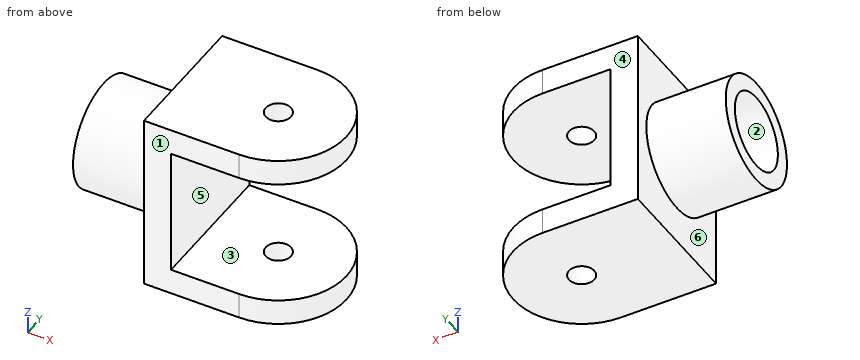
from build123d import *

# Parameters (mm, degrees)
BOSS_EXTRUDE2_DEPTH      = 11.35
BOSS_EXTRUDE2_DEPTH_BACK = 11.35
SKETCH1_R                = 1.5875
CUT_EXTRUDE1_DEPTH       = 8.08
CUT_EXTRUDE1_DEPTH_BACK  = 8.08
SKETCH3_W                = 17.175
SKETCH3_H                = 17.175
SKETCH4_R                = 6.7225
SKETCH4_R_2              = 4.7225
BOSS_EXTRUDE4_DEPTH      = 10


with BuildPart() as part:
    # Sketch1 → Boss-Extrude2 (new, two sides: drawn at the far end of the back side and taken through both)
    with BuildSketch(Plane.XY.offset(-BOSS_EXTRUDE2_DEPTH_BACK)):
        with BuildLine():
            Line((0, 8.5875), (-12, 8.5875))
            Line((-12, 8.5875), (-12, -8.5875))
            Line((-12, -8.5875), (0, -8.5875))
            ThreePointArc((0, -8.5875), (8.5875, 0), (0, 8.5875))
        make_face()
        Circle(SKETCH1_R, mode=Mode.SUBTRACT)
    extrude(amount=BOSS_EXTRUDE2_DEPTH + BOSS_EXTRUDE2_DEPTH_BACK)

    # Sketch3 → Cut-Extrude1 (cut, two sides: drawn at the far end of the back side and taken through both)
    with BuildSketch(Plane.XY.offset(-CUT_EXTRUDE1_DEPTH_BACK)):
        Rectangle(SKETCH3_W, SKETCH3_H)
    extrude(amount=CUT_EXTRUDE1_DEPTH + CUT_EXTRUDE1_DEPTH_BACK, mode=Mode.SUBTRACT)

    # Sketch4 → Boss-Extrude4 (add)
    with BuildSketch(Plane.ZY.offset(12)):
        with Locations(Location((0, 0, 0), (0, 0, 270))):
            Circle(SKETCH4_R)
        with Locations(Location((0, 0, 0), (0, 0, 270))):
            Circle(SKETCH4_R_2, mode=Mode.SUBTRACT)
    extrude(amount=BOSS_EXTRUDE4_DEPTH)


solid = part.part
The listing builds one solid part. Answer for the finished solid, in the listing's coordinates (mm). Face numbers are marked on the shaded views. A direction names the side the tool comes from. Round coordinates to 2 decimals unless told otherwise and drop trailing zeros. Order: outer loops, then holes, each group sorted by start corner. A loop starts at its lowest first (then second) coordinate and runs counter-clockwise, first axis right, second up. Notation, with made-up numbers: M 39.5,-15.75 L 48.5,-15.75 A18 cw 48.5,6.25 Z; hole C 45,65 d4. An arc over 180 degrees is marked long. Answer in a Markdown table with one row per item. Add a question column.
1) The part is cut by section C-C on z = 0. Determine the outline of the cut face in (x, y), plus the area to 3 significant figures.
2) The part is cut by section D-D on z = -8.75. Determine the outline of the cut face in (x, y) (1 decimal).
3) Which of the six approach directions +Z, -Z, +X, -X, +Y, -Y give full straight-line access (tool end or side, diameter ignored) to the marked faces 4, 5 and 6?
4) The part is cut by section A-A on x = -4.5. Determine the outline of the cut face in (y, z).
5) The part is cut by section B-B on y = 0. Determine the outline of the cut face in (x, z), plus the area to 3 significant figures.
6) Flat-ended cylindrical pins translate along their axes: pin 1 Ø5 at (x, z) = (-13, 4) entering from +Y; pin 2 Ø8.5 at (y, z) = (0, 0) entering from -X; pin 3 Ø5 at (y, z) = (-0.5, -2) entering from +X. Find the tip coordinate at first contact, or state that the pin passes through.
7) Determine the mould class of the marked faces 1, 2 and 3 for opening direction Y: pulls with the +Y half, pulls with the -Y half, needs draft (parallel to the pull), parting line crosses it, or undercut.
8) Consider line 1 along Y through (x, z) = (0, 10.45); line 2 along X through (y, z) = (0, 9.45); line 3 along Z through (x, y) = (-3, -6.25). Determine where each line is inside the solid, lowest interval first. Write a range as from..to.
Findings below:
| question | item | result |
|---|---|---|
| 1 | outline | M -22,-6.72 L -12,-6.72 L -12,-8.59 L -8.59,-8.59 L -8.59,8.59 L -12,8.59 L -12,6.72 L -22,6.72 L -22,4.72 L -12,4.72 L -12,-4.72 L -22,-4.72 Z |
| 1 | area | 98.6 mm² |
| 2 | outline | M -12,-8.6 L 0,-8.6 A8.6 ccw 0,8.6 L -12,8.6 Z; hole C 0,0 d3.2 |
| 3 | face 4 | +Z, -Z, +X, -X, +Y |
| 3 | face 5 | +X, +Y, -Y |
| 3 | face 6 | -X |
| 4 | outline | M -8.59,-11.35 L 8.59,-11.35 L 8.59,-8.08 L -8.59,-8.08 Z; M -8.59,8.08 L 8.59,8.08 L 8.59,11.35 L -8.59,11.35 Z |
| 5 | outline | M -22,-6.72 L -12,-6.72 L -12,-11.35 L -1.59,-11.35 L -1.59,-8.08 L -8.59,-8.08 L -8.59,8.08 L -1.59,8.08 L -1.59,11.35 L -12,11.35 L -12,6.72 L -22,6.72 L -22,4.72 L -12,4.72 L -12,-4.72 L -22,-4.72 Z; M 1.59,-11.35 L 8.59,-11.35 L 8.59,-8.08 L 1.59,-8.08 Z; M 1.59,8.08 L 8.59,8.08 L 8.59,11.35 L 1.59,11.35 Z |
| 5 | area | 209 mm² |
| 6 | pin 1 | stops at y = 8.59 |
| 6 | pin 2 | stops at x = -12 |
| 6 | pin 3 | stops at x = -8.59 |
| 7 | face 1 | pulls with the -Y half |
| 7 | face 2 | undercut |
| 7 | face 3 | needs draft |
| 8 | line 1 | y = -8.59..-1.59, 1.59..8.59 |
| 8 | line 2 | x = -12..-1.59, 1.59..8.59 |
| 8 | line 3 | z = -11.35..-8.08, 8.08..11.35 |
